The listing builds one solid part. Answer for the finished solid, in the listing's coordinates (mm). Face numbers are marked on the shaded views. A direction names the side the tool comes from. Coordinates: 2 decimals unless noted, no trailing zeros. Loops run counter-clockwise (first coordinate to the right, second up) from the corner with the lowest first, then second, coordinate; pieces in that order, holes last. Notation, with made-up numbers: (39.25, 79) - (83.25, 79) arc R5 cw to (83.25, 86) - close; hole circle Ø3 at (-24.5, 31). An arc over 180 degrees is marked (long way). Return JSON: item names as keys, results as strings. Group by question number.
1. Which of the six approach directions +Z, -Z, +X, -X, +Y, -Y give full straight-line access (tool end or side, diameter ignored) to the marked faces 4, 5 and 6?
2. Section A-A (x = 16.9) is taken. Write down the section's boundary in (y, z), and give its area (3 significant figures).
3. The mould has two halves that part along X. Classify the marked faces 1, 2 and 3: pulls with the +X half, pulls with the -X half, needs draft (parallel to the pull), parting line crosses it, or undercut.
4. Find the intervals of material crossed by line 1 along X through (y, z) = (-1.2, -10); line 2 along X through (y, z) = (-1.45, -8); line 3 along X through (y, z) = (-1.6, -6.5), in increasing order.
5. Section C-C (z = -10) is taken. Write down the section's boundary in (x, y), and give its area (3 significant figures).
6. Each of these flat-tipped pins is pushed along its axis until it touches: P1, Ø2, axis at x = 0, z = -8, coming from the -Y side; P2, Ø1.5, axis at x = -16.9, z = -10, coming from the -Y side; P3, Ø2, axis at x = 0.5, z = -0.5, coming from the +Y side. Where does it stop, or does it pass through?
7. Section B-B (y = -1) is taken. Write down the section's boundary in (x, z).
8. Section D-D (y = 1.3) is taken. Write down the section's boundary in (x, z), and give its area (3 significant figures).
```python
from build123d import *

# Parameters (mm, degrees)
SKETCH_1_W          = 10
SKETCH_1_H          = 16.3
SKETCH_1_R          = 2.5
EXTRUDE_1_DEPTH     = 2
SKETCH_3_W          = 10
SKETCH_3_H          = 16.3
SKETCH_3_R          = 0.95
SKETCH_3_W_2        = 1.5
SKETCH_3_H_2        = 1
EXTRUDE_2_DEPTH     = 3
SKETCH_4_W          = 14.3
SKETCH_4_H          = 16.3
EXTRUDE_3_DEPTH     = 5
SKETCH_5_R          = 0.95
CUT_EXTRUDE_1_DEPTH = 5
SKETCH_6_W          = 5
SKETCH_6_H          = 10
CUT_EXTRUDE_2_DEPTH = 3


with BuildPart() as part:
    # 草图1 → 凸台-拉伸1 (new body)
    with BuildSketch(Plane(origin=(0, 0, 0), x_dir=(1, 0, 0), z_dir=(0, 1, 0))):
        with Locations((0, 3.85)):
            Rectangle(SKETCH_1_W, SKETCH_1_H)
        with Locations(Location((0, 8, 0), (0, 0, 270))):
            Circle(SKETCH_1_R, mode=Mode.SUBTRACT)
        with BuildLine():
            Line((-1.75, 2.25), (1.75, 2.25))
            ThreePointArc((1.75, 2.25), (2.457106781, 1.957106781), (2.75, 1.25))
            Line((2.75, 1.25), (2.75, -1.25))
            ThreePointArc((2.75, -1.25), (2.457106781, -1.957106781), (1.75, -2.25))
            Line((1.75, -2.25), (-1.75, -2.25))
            ThreePointArc((-1.75, -2.25), (-2.457106781, -1.957106781), (-2.75, -1.25))
            Line((-2.75, -1.25), (-2.75, 1.25))
            ThreePointArc((-2.75, 1.25), (-2.457106781, 1.957106781), (-1.75, 2.25))
        make_face(mode=Mode.SUBTRACT)
    extrude(amount=EXTRUDE_1_DEPTH)

    # 草图3 → 凸台-拉伸2 (add)
    with BuildSketch(Plane.XZ):
        with Locations((0, -3.85)):
            Rectangle(SKETCH_3_W, SKETCH_3_H)
        with Locations(Location((0, -8, 0), (0, 0, 270))):
            Circle(SKETCH_3_R, mode=Mode.SUBTRACT)
        with Locations((-2, 0)):
            Rectangle(SKETCH_3_W_2, SKETCH_3_H_2, mode=Mode.SUBTRACT)
        with Locations((2, 0)):
            Rectangle(SKETCH_3_W_2, SKETCH_3_H_2, mode=Mode.SUBTRACT)
    extrude(amount=EXTRUDE_2_DEPTH)

    # 草图4 → 凸台-拉伸3 (add)
    with BuildSketch(Plane.XZ.offset(3)):
        with Locations((12.15, -3.85)):
            Rectangle(SKETCH_4_W, SKETCH_4_H)
        with Locations((-12.15, -3.85)):
            Rectangle(SKETCH_4_W, SKETCH_4_H)
    extrude(amount=-EXTRUDE_3_DEPTH)

    # 草图5 → 切除-拉伸1 (cut)
    with BuildSketch(Plane(origin=(0, 2, 0), x_dir=(1, 0, 0), z_dir=(0, 1, 0))):
        with Locations(Location((-16.9, 10, 0), (0, 0, 270))):
            Circle(SKETCH_5_R)
        with Locations(Location((16.9, 10, 0), (0, 0, 270))):
            Circle(SKETCH_5_R)
    extrude(amount=-CUT_EXTRUDE_1_DEPTH, mode=Mode.SUBTRACT)

    # 草图6 → 切除-拉伸2 (cut)
    with BuildSketch(Plane.XZ.offset(3)):
        with Locations((-8.5, -2.7)):
            Rectangle(SKETCH_6_W, SKETCH_6_H)
        with Locations((8.5, -2.7)):
            Rectangle(SKETCH_6_W, SKETCH_6_H)
    extrude(amount=-CUT_EXTRUDE_2_DEPTH, mode=Mode.SUBTRACT)


solid = part.part
```
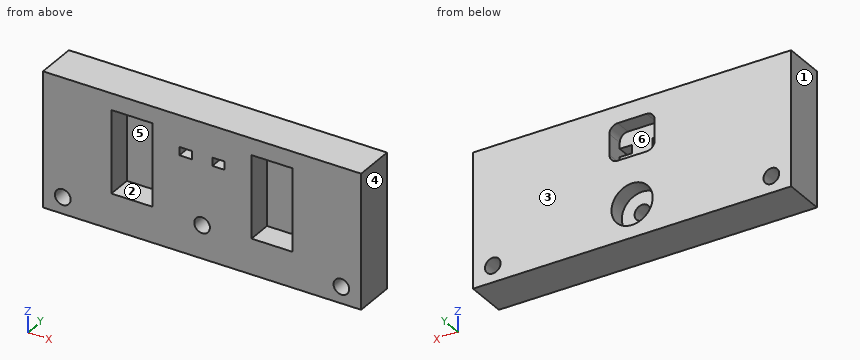
The answers:
{
 "1": {"face 4": "+Z, -Z, +X, +Y, -Y", "face 5": "-Y", "face 6": "+Y"},
 "2": {"outline": "(-3, -12) - (2, -12) - (2, -10.95) - (-3, -10.95) - close; (-3, -9.05) - (2, -9.05) - (2, 4.3) - (-3, 4.3) - close", "area": "72.0 mm2"},
 "3": {"face 1": "pulls with the -X half", "face 2": "undercut", "face 3": "needs draft"},
 "4": {"line 1": "x = -19.3 to -17.85, -15.95 to 15.95, 17.85 to 19.3", "line 2": "x = -19.3 to -0.95, 0.95 to 19.3", "line 3": "x = -19.3 to -11, -6 to 6, 11 to 19.3"},
 "5": {"outline": "(-19.3, -3) - (-17.85, -3) - (-17.85, 2) - (-19.3, 2) - close; (-15.95, -3) - (15.95, -3) - (15.95, 2) - (1.5, 2) - (1.5, 0) - (-1.5, 0) - (-1.5, 2) - (-15.95, 2) - close; (17.85, -3) - (19.3, -3) - (19.3, 2) - (17.85, 2) - close", "area": "168 mm2"},
 "6": {"P1": "stops at y = -3", "P2": "passes through", "P3": "stops at y = 0"},
 "7": {"outline": "(-19.3, -12) - (19.3, -12) - (19.3, 4.3) - (-19.3, 4.3) - close; hole circle Ø1.9 at (-16.9, -10); hole (-11, -7.7) - (-6, -7.7) - (-6, 2.3) - (-11, 2.3) - close; hole (-2.75, -0.5) - (-1.25, -0.5) - (-1.25, 0.5) - (-2.75, 0.5) - close; hole circle Ø1.9 at (0, -8); hole (1.25, -0.5) - (2.75, -0.5) - (2.75, 0.5) - (1.25, 0.5) - close; hole (6, -7.7) - (11, -7.7) - (11, 2.3) - (6, 2.3) - close; hole circle Ø1.9 at (16.9, -10)"},
 "8": {"outline": "(-19.3, -12) - (19.3, -12) - (19.3, 4.3) - (-19.3, 4.3) - close; hole circle Ø1.9 at (-16.9, -10); hole (-2.75, -1.25) arc R1 ccw to (-1.75, -2.25) - (1.75, -2.25) arc R1 ccw to (2.75, -1.25) - (2.75, 1.25) arc R1 ccw to (1.75, 2.25) - (-1.75, 2.25) arc R1 ccw to (-2.75, 1.25) - close; hole circle Ø5 at (0, -8); hole circle Ø1.9 at (16.9, -10)", "area": "580 mm2"}
}
